Model file for the job. Use its own axes, mm. A direction names the side the tool comes from. Round coordinates to 2 decimals unless told otherwise and drop trailing zeros. Loops run counter-clockwise (first coordinate to the right, second up) from the corner with the lowest first, then second, coordinate; pieces in that order, holes last. Notation, with made-up numbers: M -3.5,46 L 39.5,46 A21 ccw 39.5,83 Z; hole C 30,63 d6. An arc over 180 degrees is marked long. Use a Markdown table: item, result. Add a question column.
Item 1: Saw through at B-B on y = -11. Write the cut outline in (x, z).
Item 2: Tool access for faces 1 (the cylindrical face through (1.578, -37.517, 34.536)), 2 (the cylindrical face through (1.578, -36.363, 36.456)), 3 (the flat face through (-2, 0, 20)), 4 (the cylindrical face through (1.578, -2.015, 0.894)), 5 (the cylindrical face through (1.578, 0.104, -0.006)): list every direction of +Z, -Z, +X, -X, +Y, -Y with a clear straight run to the whole face (end or side of a thin tool).
Item 3: Saw through at D-D on y = -59. Write the cut outline in (x, z), then the cut area to 3 significant figures.
Item 4: Saw through at A-A on z = 27.5. Write the cut outline in (x, y).
Item 5: Wall check: L1, parallel to Y at x = 16, z = 24.5; L2, parallel to Y at x = 55, z = 11; L3, parallel to Z at x = -13, y = -10. Give the ranges that are in metal, low to high. Write a range as from..to.
Item 6: Saw through at C-C on z = 8. Write the cut outline in (x, y).
Item 7: Pin check, flat tips, straight feed: P1, Ø0.6, axis at x = 50.5, z = 24, coming from the +Y side; P2, Ø10, axis at x = -84, y = -24, coming from the +Z side; P3, Ø2, axis at x = 2.5, y = -2, coming from the +Z side; P4, Ø8, axis at y = -22, z = 29.5, coming from the -X side. Stop position of each tip, or through.
```python
from build123d import *

# Parameters (mm, degrees)
F1_DEPTH  = 112.7125
F2_T      = -1.524
F5_DEPTH  = 225.425
F7_DEPTH  = 225.425
F8_R      = 51.8099901909
F9_DEPTH  = 225.425
F14_W     = 1.27
F14_H     = 1.8664713708
F15_DEPTH = 225.425
F17_DEPTH = 225.425
F18_W     = 0.5953125
F18_H     = 31.75
F19_DEPTH = 225.425
F21_DEPTH = 225.425
F23_DEPTH = 225.425
F24_R     = 0.508
F25_R     = 6.35
F26_R     = 0.254


with BuildPart() as f1:
    # F0 (on Right) → F1 (new body, symmetric)
    with BuildSketch(Plane.YZ):
        with BuildLine():
            Line((-72.136, 14.4276117903), (-26.3105725372, -25.4078245579))
            Line((-26.3105725372, -25.4078245579), (0, 0))
            Line((0, 0), (0, 37.338))
            ThreePointArc((0, 37.338), (-36.8647965725, 36.3151722047), (-68.7392263709, 17.7657752319))
            Line((-68.7392263709, 17.7657752319), (-72.136, 14.4276117903))
        make_face()
    extrude(amount=F1_DEPTH, both=True)

    # F2
    f2_openings = [f1.faces().sort_by_distance(p)[0] for p in [
        (0, -49.223286, -5.490106),
        (-112.7125, -29.609995, 11.681685),
        (112.7125, -29.609995, 11.681685),
    ]]
    offset(amount=F2_T, openings=f2_openings)

    # F4 (on face) → F5 (join, through all)
    with BuildSketch(Plane(origin=(-112.7125, 0, 0), x_dir=(0, -1, 0), z_dir=(-1, 0, 0))):
        Polygon((69.0653059094, 11.7582981414), (70.9822682431, 13.424688075), (69.170655641, 15.2050419106), (67.2536933072, 13.5386519769), align=None)
    extrude(amount=-F5_DEPTH)

    # F6 (on face) → F7 (join, through all)
    with BuildSketch(Plane(origin=(-112.7125, 0, 0), x_dir=(0, -1, 0), z_dir=(-1, 0, 0))):
        Polygon((27.5549826692, -20.9733491998), (25.6380203354, -22.6397391335), (27.4651434283, -24.4041713944), (29.382105762, -22.7377814608), align=None)
    extrude(amount=-F7_DEPTH)

    # F8 (on face) → F9 (cut, through all)
    with BuildSketch(Plane(origin=(-112.7125, 0, 0), x_dir=(0, -1, 0), z_dir=(-1, 0, 0))):
        with Locations((76.7665722185, -37.1750323717)):
            Circle(F8_R)
    extrude(amount=-F9_DEPTH, mode=Mode.SUBTRACT)

    # F10 (on face) + F11 (on face) + F12 (on face) + F13 (on face) + F14 (on face) → F15 (join, through all)
    with BuildSketch(Plane(origin=(-112.7125, 0, 0), x_dir=(0, -1, 0), z_dir=(-1, 0, 0))):
        Polygon((23.17140416, -20.2577555812), (24.0849657065, -21.1399717116), (25.5666650167, -19.8519501518), (24.530017001, -18.8508707997), align=None)
    with BuildSketch(Plane(origin=(-112.7125, 0, 0), x_dir=(0, -1, 0), z_dir=(-1, 0, 0))):
        Polygon((23.6164554546, -17.9686546692), (25.5666650167, -19.8519501518), (26.4488811472, -18.9383886054), (24.498671585, -17.0550931227), align=None)
    with BuildSketch(Plane(origin=(-112.7125, 0, 0), x_dir=(0, -1, 0), z_dir=(-1, 0, 0))):
        Polygon((65.7138225954, 15.0519527371), (67.6307849291, 16.7183426707), (66.724978628, 17.6085195885), (64.8080162943, 15.9421296549), align=None)
    with BuildSketch(Plane(origin=(-112.7125, 0, 0), x_dir=(0, -1, 0), z_dir=(-1, 0, 0))):
        Polygon((13.0308709947, -10.4651565328), (13.9444325411, -11.3473726633), (15.303045382, -9.9404878818), (16.2166069285, -10.8227040123), (17.098823059, -9.9091424658), (15.2716999661, -8.1447102049), align=None)
    with BuildSketch(Plane(origin=(-112.7125, 0, 0), x_dir=(0, -1, 0), z_dir=(-1, 0, 0))):
        Polygon((1.524, 23.2821790422), (1.524, 22.0121790422), (4.7498, 22.0121790422), (4.7498, 24.5521790422), (3.4798, 24.5521790422), (3.4798, 23.2821790422), align=None)
        with Locations((4.1148, 35.7724147276)):
            Rectangle(F14_W, F14_H)
    extrude(amount=-F15_DEPTH)

    # F16 (on face) → F17 (join, through all)
    with BuildSketch(Plane(origin=(-112.7125, 0, 0), x_dir=(0, -1, 0), z_dir=(-1, 0, 0))):
        Polygon((-0.5953125, 37.2036794522), (-0.5953125, -0.252695164), (26.1530440412, -26.0832828204), (26.3105725372, -25.4078245579), (0, 0), (0, 37.338), align=None)
    extrude(amount=-F17_DEPTH)

    # F18 (on face) → F19 (cut, through all)
    with BuildSketch(Plane(origin=(-112.7125, 0, 0), x_dir=(0, -1, 0), z_dir=(-1, 0, 0))):
        with Locations((-0.29765625, 20.2341790422)):
            Rectangle(F18_W, F18_H)
    extrude(amount=-F19_DEPTH, mode=Mode.SUBTRACT)

    # F20 (on face) → F21 (cut, through all)
    with BuildSketch(Plane(origin=(-112.7125, 0, 0), x_dir=(0, -1, 0), z_dir=(-1, 0, 0))):
        Polygon((3.2705379083, -3.1583217457), (2.8569990972, -3.5865537206), (21.6992059923, -21.7822614118), (22.1127448035, -21.3540294369), align=None)
    extrude(amount=-F21_DEPTH, mode=Mode.SUBTRACT)

    # F22 (on face) → F23 (cut, through all)
    with BuildSketch(Plane(origin=(-112.7125, 0, 0), x_dir=(0, -1, 0), z_dir=(-1, 0, 0))):
        with BuildLine():
            Line((25.6380203354, -22.6397391335), (24.0849657065, -21.1399717116))
            ThreePointArc((24.0849657065, -21.1399717116), (24.2715109837, -22.5007997067), (25.6380203354, -22.6397391335))
        make_face()
    extrude(amount=-F23_DEPTH, mode=Mode.SUBTRACT)

    # F24
    f24_edges = [f1.edges().sort_by_distance(p)[0] for p in [
        (0, -72.136, 14.427612),
        (0, 0.595312, 37.203679),
        (0, -26.153044, -26.083283),
    ]]
    fillet(f24_edges, radius=F24_R)

    # F25
    f25_edges = [f1.edges().sort_by_distance(p)[0] for p in [
        (0, -1.524, 0.6469),
        (0, 0.595313, -0.252695),
    ]]
    fillet(f25_edges, radius=F25_R)

    # F26
    f26_edges = [f1.edges().sort_by_distance(p)[0] for p in [
        (0, -27.554983, -20.973349),
        (0, -67.567953, 13.811833),
    ]]
    fillet(f26_edges, radius=F26_R)


solid = f1.part
```
Entries:
| question | item | result |
|---|---|---|
| 1 | outline | M -112.71,-10.62 L 112.71,-10.62 L 112.71,-8.5 L -112.71,-8.5 Z; M -112.71,37.44 L 112.71,37.44 L 112.71,38.97 L -112.71,38.97 Z |
| 2 | face 1 | +X, -X |
| 2 | face 2 | +Z, +X, -X |
| 2 | face 3 | +X, -X, +Y |
| 2 | face 4 | +X, -X, -Y |
| 2 | face 5 | -Z, +X, -X, +Y |
| 3 | outline | M -112.71,23.97 L 112.71,23.97 L 112.71,25.83 L -112.71,25.83 Z |
| 3 | area | 420 mm2 |
| 4 | outline | M -112.71,-56.5 L 112.71,-56.5 L 112.71,-53.58 L -112.71,-53.58 Z; M -112.71,-1.52 L 112.71,-1.52 L 112.71,0 L -112.71,0 Z |
| 5 | L1 | -60.86..-58.25, -4.75..-3.48, -1.52..0 |
| 5 | L2 | -1.52..0 |
| 5 | L3 | -9.66..-7.54, 37.36..38.89 |
| 6 | outline | M -112.71,-1.52 L 112.71,-1.52 L 112.71,0 L -112.71,0 Z |
| 7 | P1 | y = 0 |
| 7 | P2 | z = 39.12 |
| 7 | P3 | z = 37.95 |
| 7 | P4 | through |
